Design review of the part built by this model. Coordinates are the model's own, in mm. A direction names the side the tool comes from. Give positions to 0.01 mm unless a question says otherwise; leave off trailing zeros. Write each loop counter-clockwise with the first axis right and the second up, starting at its lowest first coordinate (ties: lowest second). Pieces come first, ordered by that corner, then holes. Notation, with made-up numbers: M 78,61 L 109,61 A29 cw 109,91 Z; hole C 56,35 d5. An arc over 180 degrees is marked long. Use a Markdown table: item, result. Add a question column.
```python
from build123d import *

# Parameters (mm, degrees)
F2_DEPTH = 25.4
F3_W     = 6.096
F3_H     = 50.8
F4_DEPTH = 25.4
F5_R     = 5.08
F6_R     = 3.175
F7_DEPTH = 6.097
F8_R     = 3.175
F9_DEPTH = 6.097


# Not quite as in the source:
# - a feature names something its author has since deleted; it is built from what else it names


with BuildPart() as f2:
    # F1 (on Front) → F2 (new body)
    with BuildSketch(Plane.XZ):
        with BuildLine():
            ThreePointArc((-4.1881381368, 58.1348573723), (-17.2625408115, 33.1930369346), (-45.2129217657, 29.7563791738))
            ThreePointArc((-45.2129217657, 29.7563791738), (-47.3496102258, 30.6565141034), (-49.4112893939, 31.7172494495))
            Line((-49.4112893939, 31.7172494495), (-52.5301234092, 26.1859408896))
            ThreePointArc((-52.5301234092, 26.1859408896), (-50.0367693734, 24.903108528), (-47.4527005825, 23.8145031357))
            ThreePointArc((-47.4527005825, 23.8145031357), (-41.0907281326, 22.0513224192), (-34.5157381367, 21.4571791316))
            Line((-34.5157381367, 21.4571791316), (1.9167693099, 21.4571791316))
            Line((1.9167693099, 21.4571791316), (1.9167693099, 62.3678327477))
            ThreePointArc((1.9167693099, 62.3678327477), (-10.1232383217, 85.5255128665), (-34.5157381367, 94.8123791316))
            ThreePointArc((-34.5157381367, 94.8123791316), (-41.4558425944, 94.1497939431), (-48.145199434, 92.1859777376))
            ThreePointArc((-48.145199434, 92.1859777376), (-50.3725422349, 91.2075489816), (-52.5301234092, 90.0836173735))
            Line((-52.5301234092, 90.0836173735), (-49.4112893939, 84.5523088136))
            ThreePointArc((-49.4112893939, 84.5523088136), (-47.6272506666, 85.4816539244), (-45.7855281567, 86.2906871202))
            ThreePointArc((-45.7855281567, 86.2906871202), (-17.5160993904, 83.2500255818), (-4.1881381368, 58.1348573723))
        make_face()
    extrude(amount=F2_DEPTH)

    # F3 (on offset) → F4 (join)
    with BuildSketch(Plane.XY.offset(30.353)):
        with Locations((-1.1312306901, -12.7)):
            Rectangle(F3_W, F3_H)
    extrude(amount=F4_DEPTH)

    # F5
    f5_edges = [f2.edges().sort_by_distance(p)[0] for p in [
        (1.916769, -12.7, 62.367833),
        (-1.131231, -38.1, 55.753),
        (-1.131231, -38.1, 30.353),
        (-1.131231, 12.7, 30.353),
        (-1.131231, 12.7, 55.753),
    ]]
    fillet(f5_edges, radius=F5_R)

    # F6 (on face) → F7 (cut, through all)
    with BuildSketch(Plane(origin=(-4.1792306901, 0, 0), x_dir=(0, -1, 0), z_dir=(-1, 0, 0))):
        with Locations((-3.81, 43.053)):
            Circle(F6_R)
    extrude(amount=-F7_DEPTH, mode=Mode.SUBTRACT)

    # F8 (on face) → F9 (cut, through all)
    with BuildSketch(Plane(origin=(-4.1792306901, 0, 0), x_dir=(0, -1, 0), z_dir=(-1, 0, 0))):
        with Locations((29.21, 43.053)):
            Circle(F8_R)
    extrude(amount=-F9_DEPTH, mode=Mode.SUBTRACT)


solid = f2.part
```
(1) Add section A-A on y = 3.81. Give the boundary of the cut face in (x, z), then the cut area to 3 significant figures.
(2) Add section D-D on y = -23. Give the boundary of the cut face in (x, z).
(3) Machinability: for faces 4 (the flat face through (-1, 4, 55.753)), 5 (the flat face through (-1, 4, 30.353)), 6 (the flat face through (-50.993, -12.522, 87.357)), which of the approach directions +Z, -Z, +X, -X, +Y, -Y give a long, thin tool a straight path to every point of the face, cutting with its end or side? Answer none if there is none.
(4) Add section C-C on z = 41. Give the boundary of the cut face in (x, y).
(5) For pin 1 (4 mm diameter, centred on y = -7.5, z = 65.5, fed in from +X); pin 2 (3 mm diameter, centred on y = 3.5, z = 55.5, fed in from -X); pin 3 (1.5 mm diameter, centred on x = -18.5, z = 81, fed in from -Y); pin 4 (1.8 mm diameter, centred on x = -2, y = -28.5, fed in from -Z), all flat-tipped, find the tip position at first contact; note any pin that passes through.
(6) The part is to be moulded in two halves that separate along Z. For faces 1 (the flat face through (-50.95, -12.52, 28.99)), 2 (the flat face through (-1, -29, 30.353)), 3 (the cylindrical face through (-1.089, 11.172, 54.304)), say which applies: released by +Z, released by -Z, zero draft, split by the parting line, or undercut.
(7) Add section B-B on x = -43. Give the boundary of the cut face in (y, z), then the cut area to 3 significant figures.
(8) Wall thickness on L1, parallel to Z at x = 0, y = -29; L2, parallel to X at y = 8, z = 51.5; L3, parallel to Z at x = -26, y = -23: over which ranges is each line inside the solid? List them lowest first.
From the geometry:
| question | item | result |
|---|---|---|
| 1 | outline | M -4.18,30.35 L 1.92,30.35 L 1.92,39.88 L -4.18,39.88 Z; M -4.18,46.23 L 1.92,46.23 L 1.92,55.75 L -4.18,55.75 Z |
| 1 | area | 116 mm^2 |
| 2 | outline | M -52.53,26.19 A36.68 ccw -34.52,21.46 L 1.92,21.46 L 1.92,62.06 A5.08 ccw 1.88,62.69 A36.68 ccw -52.53,90.08 L -49.41,84.55 A30.33 cw long -49.41,31.72 Z |
| 3 | face 4 | +Z, +X, -X, +Y |
| 3 | face 5 | -Z, +X, -X, +Y |
| 3 | face 6 | -X, +Y, -Y |
| 4 | outline | M -9.49,-25.4 L -4.18,-25.4 L -4.18,-26.79 L 1.92,-26.79 L 1.92,1.39 L -4.18,1.39 L -4.18,0 L -9.49,0 Z; M -4.18,-38.1 L 1.92,-38.1 L 1.92,-31.63 L -4.18,-31.63 Z; M -4.18,6.23 L 1.92,6.23 L 1.92,12.7 L -4.18,12.7 Z |
| 5 | pin 1 | stops at x = 1.77 |
| 5 | pin 2 | stops at x = -4.18 |
| 5 | pin 3 | passes through |
| 5 | pin 4 | stops at z = 30.35 |
| 6 | face 1 | undercut |
| 6 | face 2 | released by -Z |
| 6 | face 3 | released by +Z |
| 7 | outline | M -25.4,22.45 L 0,22.45 L 0,29.02 L -25.4,29.02 Z; M -25.4,87.25 L 0,87.25 L 0,93.82 L -25.4,93.82 Z |
| 7 | area | 334 mm^2 |
| 8 | L1 | z = 30.35 to 39.88, 46.22 to 55.75 |
| 8 | L2 | x = -4.18 to 1.92 |
| 8 | L3 | z = 21.46 to 29.03, 87.24 to 93.81 |
